Here's how the part is built. I have some questions about the finished solid (model axes, mm). A direction names the side the tool comes from. Give positions to 0.01 mm unless a question says otherwise; leave off trailing zeros. Write each loop counter-clockwise with the first axis right and the second up, starting at its lowest first coordinate (ties: lowest second). Pieces come first, ordered by that corner, then holes. Notation, with made-up numbers: (47, 37.5) - (75, 37.5) arc R29 cw to (75, 75.5) - close; hole circle Ø5 at (13.5, 60.5). An arc over 180 degrees is marked (long way). Write each question's results on one line, items separated by ' | '. Start each with the question number.
Item 1: Suppose I cut it at D-D on x = -17. List the corners of the cut face in (y, z) for me, then the cut area to 3 significant figures.
Item 2: Please list where these lines run through material, in increasing order: line 1 along Y through (x, z) = (0, 8.2) (3 decimals); line 2 along Z through (x, y) = (-6, 12); line 3 along Y through (x, z) = (10, 18).
Item 3: Suppose I cut it at C-C on z = 23.5. List the corners of the cut face in (x, y) for me, then the cut area to 3 significant figures.
Item 4: Which directions (+Z, -Z, +X, -X, +Y, -Y) give clear straight access to the entire face, cutting with the end or side of a thin tool? Please do faces 1 (the cylindrical face through (-24, 0, 17)), 2 (the flat face through (19, 0, 25)).
Item 5: We'd pull the mould along X, two halves only. Please class faces 3 (the cylindrical face through (23.846, 7.509, 7.465)), 4 (the flat face through (-10, -16, 25)), 5 (the cylindrical face through (-6.05, -4.64, 7.46)): +X half, -X half, draft (parallel to the pull), parting line (faces both ways), or undercut.
Item 6: Suppose I cut it at A-A on x = 0. List the corners of the cut face in (y, z) for me (3 decimals), then the cut area to 3 significant figures.
Item 7: Suppose I cut it at B-B on y = 0. List the corners of the cut face in (x, z) for me (3 decimals), then the cut area to 3 significant figures.
Item 8: Will these pins go through, and if not, where does the flat tip stop? P1, Ø9, axis at x = 0, y = 0, coming from the +Z side; P2, Ø8, axis at y = 3, z = 18.5, coming from the +X side; P3, Ø6, axis at y = -9.5, z = 7.5, coming from the -X side; P4, Ø12, axis at x = 4.5, z = 13.5, coming from the +Y side.
```python
from build123d import *

# Parameters (mm, degrees)
DRIVERDISKBASESKETCH001_R   = 25
DRIVERDISKBASESKETCH001_R_2 = 7.625
PAD_DEPTH                   = 5
DRIVERSHAFTSKETCH_R         = 5
PAD004_DEPTH                = 20
DRIVERDISKPOLAR_COUNT       = 6


with BuildPart() as part:
    # DriverDiskBaseSketch001 → Pad (new body)
    with BuildSketch(Plane.XY):
        Circle(DRIVERDISKBASESKETCH001_R)
        Circle(DRIVERDISKBASESKETCH001_R_2, mode=Mode.SUBTRACT)
    extrude(amount=PAD_DEPTH)

    # DriverShaftSketch → Pad004 (join)
    with BuildSketch(Plane.XY):
        with Locations((-19, 0)):
            Circle(DRIVERSHAFTSKETCH_R)
    pad004 = extrude(amount=PAD004_DEPTH)

    # DriverDiskPolar: Pad004 ×6 about axis
    driverdiskpolar_axis = Axis((0, 0, 0), (0, 0, 1))
    for i in range(1, DRIVERDISKPOLAR_COUNT):
        add(pad004.rotate(driverdiskpolar_axis, i * 360 / DRIVERDISKPOLAR_COUNT))


with BuildPart() as part_1:
    # driverDisk placement: moved
    add(part.part.moved(Location((0, 0, 5))))


solid = part_1.part
```
Checked values:
1) outline: (-18.33, 5) - (18.33, 5) - (18.33, 10) - (4.58, 10) - (4.58, 25) - (-4.58, 25) - (-4.58, 10) - (-18.33, 10) - close | area: 321 mm^2
2) line 1: y = -25 to -7.625, 7.625 to 25 | line 2: z = 5 to 10 | line 3: y = -21.43 to -11.48, 11.48 to 21.43
3) outline: circle Ø10 at (-19, 0); circle Ø10 at (-9.5, -16.45); circle Ø10 at (-9.5, 16.45); circle Ø10 at (9.5, -16.45); circle Ø10 at (9.5, 16.45); circle Ø10 at (19, 0) | area: 471 mm^2
4) face 1: +Z | face 2: +Z, +X, -X, +Y, -Y
5) face 3: parting line | face 4: draft | face 5: undercut
6) outline: (-25, 5) - (-7.625, 5) - (-7.625, 10) - (-25, 10) - close; (7.625, 5) - (25, 5) - (25, 10) - (7.625, 10) - close | area: 174 mm^2
7) outline: (-25, 5) - (-7.625, 5) - (-7.625, 10) - (-14, 10) - (-14, 25) - (-24, 25) - (-24, 10) - (-25, 10) - close; (7.625, 5) - (25, 5) - (25, 10) - (24, 10) - (24, 25) - (14, 25) - (14, 10) - (7.625, 10) - close | area: 474 mm^2
8) P1: passes through | P2: stops at x = 24 | P3: stops at x = -24.14 | P4: stops at y = 25
